CAD build for the part. Positions are in the model's coordinates, mm. A direction names the side the tool comes from. Round coordinates to 2 decimals unless told otherwise and drop trailing zeros. Write each loop counter-clockwise with the first axis right and the second up, starting at its lowest first coordinate (ties: lowest second). Pieces come first, ordered by that corner, then holes. Notation, with made-up numbers: (54, 88.25) -> (92, 88.25) arc R17 ccw to (92, 116.25) -> close; hole circle Ø8 at (56, -33). An arc over 180 degrees is marked (long way). Put each result on its own line as item: value. Start each with the question number.
1. Drill centre lines: line 1 (X direction, y = 2.45, z = 10.16); line 2 (Z direction, x = -19.5, y = 4.5); line 3 (Z direction, x = 0.5, y = 2.85). Where is each one in solid material? Low to high. Write a range as from..to.
2. Saw through at A-A on x = 0. List the corners of the cut face in (y, z) (3 decimals).
3. Saw through at B-B on z = -1.5. List the corners of the cut face in (x, y), and give its area (3 significant figures).
4. 3-axis set-ups, long thin cutter, end or side, ignore diameter. For faces 1 (the flat face through (12.1, 2.5, 16.25)), 2 (the cylindrical face through (-26.644, 2.576, 8.565)): which of +Z, -Z, +X, -X, +Y, -Y reach the whole face in a straight line?
5. Flat gauge pins, fed straight in: P1, Ø2, axis at y = 3.5, z = -13.5, coming from the +X side; P2, Ø1, axis at y = 3.5, z = -19.5, coming from the -X side; P3, Ø5.5, axis at x = 17.6, z = 10.16, coming from the +Y side; P4, Ø6.5, axis at x = -5, z = -0.5, coming from the +Y side. Where does each tip first touch, or does it go through?
6. Pull direction Z, two halves, no side cores. Call faces 3 (the flat face through (6, 5.08, 10)), 4 (the cylindrical face through (-20.69, 2.58, 18.81)), 5 (the flat face through (20.3, 2.5, 2.5)), 6 (the cylindrical face through (-15.45, 2.58, 7.82)): pulls with the +Z half, pulls with the -Z half, needs draft (parallel to the pull), parting line crosses it, or undercut.
7. Saw through at D-D on y = 3.75. State how many separate pieces and enclosed holes the cut face has, and give its area (3 significant figures).
8. Saw through at C-C on x = 17.5. List the corners of the cut face in (y, z), and give its area (3 significant figures).
from build123d import *

# Parameters (mm, degrees)
SKETCH2_R                   = 11
BOSS_EXTRUDE1_DEPTH         = 5.08
SKETCH2_6_R                 = 11
SKETCH2_6_R_2               = 8
BOSS_EXTRUDE2_DEPTH         = 1.778
F_1_4_0_25_DIAMETER_HOLE3_D = 6.35
FILLET3_R                   = 2.54
CIRPATTERN2_COUNT           = 3


with BuildPart() as part:
    # Sketch2 → Boss-Extrude1 (new body)
    with BuildSketch(Plane(origin=(0, 0, 0), x_dir=(1, 0, 0), z_dir=(0, 1, 0))):
        with BuildLine():
            Line((-6.428604647, 27.94), (-9.222115265, 11.588299705))
            ThreePointArc((-9.222115265, 11.588299705), (0, -14.81), (9.222115265, 11.588299705))
            Line((9.222115265, 11.588299705), (6.428604647, 27.94))
            Line((6.428604647, 27.94), (-6.428604647, 27.94))
        make_face()
        with Locations(Location((0, 0, 0), (0, 0, 270))):
            Circle(SKETCH2_R, mode=Mode.SUBTRACT)
    extrude(amount=BOSS_EXTRUDE1_DEPTH)

    # Sketch2_6 → Boss-Extrude2 (add)
    with BuildSketch(Plane(origin=(0, 0, 0), x_dir=(1, 0, 0), z_dir=(0, 1, 0))):
        with Locations(Location((0, 0, 0), (0, 0, 270))):
            Circle(SKETCH2_6_R)
        with Locations(Location((0, 0, 0), (0, 0, 270))):
            Circle(SKETCH2_6_R_2, mode=Mode.SUBTRACT)
    extrude(amount=BOSS_EXTRUDE2_DEPTH)

    # 1_4 _0.25_ Diameter Hole3 (through all)
    with Locations(Plane(origin=(0, 0, -20.32), x_dir=(0, 0, -1), z_dir=(0, -1, 0))):
        with Locations((0, 0)):
            Hole(F_1_4_0_25_DIAMETER_HOLE3_D / 2)

    # Fillet3
    fillet3_edges = [part.edges().sort_by_distance(p)[0] for p in [
        (-6.428604647, 2.54, -27.94),
        (6.428604647, 2.54, -27.94),
    ]]
    fillet(fillet3_edges, radius=FILLET3_R)

    # CirPattern2: part ×3 about axis
    cirpattern2_axis = Axis((0, 0, 0), (0, 1, 0))


with BuildPart() as part_1:
    add(part.part)
    for i in range(1, CIRPATTERN2_COUNT):
        add(part.part.rotate(cirpattern2_axis, i * 360 / CIRPATTERN2_COUNT))


solid = part_1.part
Return value:
1. line 1: x = -26.39..-20.77, -14.42..-4.22, 4.22..14.42, 20.77..26.39
1. line 2: z = 1.84..7.62, 12.7..18.93
1. line 3: z = -27.94..-23.46, -17.18..-10.99, 10.99..14.8
2. outline: (0, -27.94) -> (5.08, -27.94) -> (5.08, -23.495) -> (0, -23.495) -> close; (0, -17.145) -> (5.08, -17.145) -> (5.08, -11) -> (1.778, -11) -> (1.778, -8) -> (0, -8) -> close; (0, 8) -> (1.778, 8) -> (1.778, 11) -> (5.08, 11) -> (5.08, 14.81) -> (0, 14.81) -> close
3. outline: (-15.48, 0) -> (-7.86, 0) -> (-7.86, 1.78) -> (-10.9, 1.78) -> (-10.9, 5.08) -> (-15.48, 5.08) -> close; (7.86, 0) -> (15.48, 0) -> (15.48, 5.08) -> (10.9, 5.08) -> (10.9, 1.78) -> (7.86, 1.78) -> close
3. area: 57.4 mm^2
4. face 1: +Z, +Y, -Y
4. face 2: -X, +Y, -Y
5. P1: stops at x = 9.07
5. P2: stops at x = -7.96
5. P3: passes through
5. P4: stops at y = 1.78
6. face 3: needs draft
6. face 4: pulls with the +Z half
6. face 5: pulls with the -Z half
6. face 6: undercut
7. separate pieces: 1
7. enclosed holes: 4
7. area: 854 mm^2
8. outline: (0, 0.18) -> (5.08, 0.18) -> (5.08, 6.99) -> (0, 6.99) -> close; (0, 13.33) -> (5.08, 13.33) -> (5.08, 18.25) -> (0, 18.25) -> close
8. area: 59.6 mm^2
